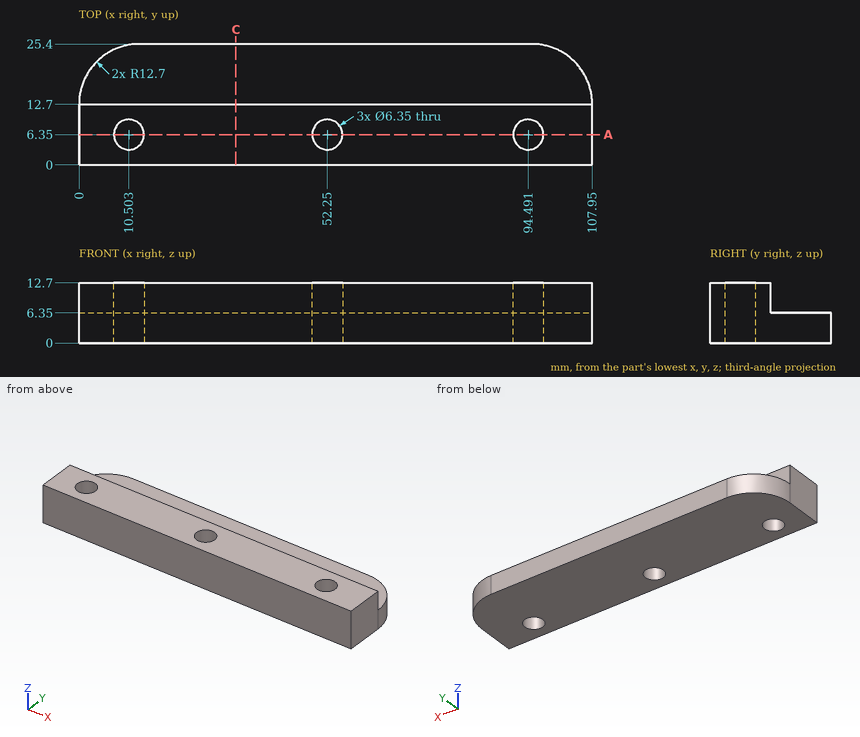
Geometry: see drawing. Coordinates: mm, zero at the bounding-box minimum. Round coordinates to 2 decimals unless told otherwise and drop trailing zeros. Loops run counter-clockwise (first coordinate to the right, second up) from the corner with the lowest first, then second, coordinate; pieces in that order, holes last. Notation, with made-up numbers: (71.5, -34.75) -> (120.5, -34.75) arc R12 ccw to (120.5, -25.75) -> close; hole circle Ø11 at (-4.75, 58). An arc over 180 degrees is marked (long way). Use one line per item in the form item = value. Start each with the question number.
Item 1: Material intervals for L1, parallel to Y at x = 52, z = 6.5 (1 decimal); L2, parallel to Y at x = 36.5, z = 11; L3, parallel to Z at x = 86.5, y = 24, sorted ascending. Write a range as from..to.
Item 2: Section query A-A on y = 6.35. Count the separate pieces of the cut face and the enclosed holes in it, then the cut area to 3 significant figures.
Item 3: Contact query for flat-ended pins moving along their axis: pin 1 Ø3 at (x, z) = (14, 7.5) entering from +Y; pin 2 Ø3 at (x, z) = (76, 10) entering from +Y; pin 3 Ø10 at (x, y) = (54.5, 18.5) entering from +Z. Output: stop coordinate, or through.
Item 4: Section query C-C on x = 33. Return the cut outline in (y, z).
Ans:
q1.L1 = 0..3.2, 9.5..12.7
q1.L2 = 0..12.7
q1.L3 = 0..6.35
q2.separate_pieces = 4
q2.enclosed_holes = 0
q2.area = 1,130 mm^2
q3.pin_1 = 25.4
q3.pin_2 = 12.7
q3.pin_3 = 6.35
q4.outline = (0, 0) -> (25.4, 0) -> (25.4, 6.35) -> (12.7, 6.35) -> (12.7, 12.7) -> (0, 12.7) -> close
